Check sheet for the modelled part. Datum: model origin and axes. Units: mm. A direction names the side the tool comes from. Round coordinates to 2 decimals unless told otherwise and drop trailing zeros. Write each loop counter-clockwise with the first axis right and the second up, starting at its lowest first coordinate (ties: lowest second). Pieces come first, ordered by that corner, then holes. Notation, with made-up numbers: (59, 0) -> (105, 0) arc R3 ccw to (105, 4) -> close; hole circle Ø10 at (51.5, 17). An arc over 180 degrees is marked (long way). One line per item, written item: value.
from build123d import *
from OCP.BRepFilletAPI import BRepFilletAPI_MakeChamfer

# Parameters (mm, degrees)
SKETCH1_R           = 2.5
SKETCH1_R_2         = 3.15
BOSS_EXTRUDE1_DEPTH = 16
SKETCH2_W           = 40
SKETCH2_H           = 20
CUT_EXTRUDE1_DEPTH  = 11
FILLET2_R           = 9
SKETCH3_R           = 6
CUT_EXTRUDE2_DEPTH  = 13.5
CUT_EXTRUDE5_DEPTH  = 67.957075802
SKETCH7_R           = 3.05
CUT_EXTRUDE6_DEPTH  = 67.957075802
CHAMFER2_SIZE       = 2
CHAMFER2_SIZE2      = 0.727940469
SKETCH10_R          = 6.1
CUT_EXTRUDE8_DEPTH  = 0.7
CHAMFER3_SIZE       = 3
CHAMFER4_SIZE       = 0.3
SKETCH11_R          = 1.65
CUT_EXTRUDE9_DEPTH  = 78.111931632
SKETCH12_R          = 3.2
CUT_EXTRUDE10_DEPTH = 3
CUT_EXTRUDE11_START = -35
CUT_EXTRUDE11_DEPTH = 43.111931632
CHAMFER5_SIZE       = 2
CHAMFER5_SIZE2      = 0.727940469
CUT_EXTRUDE12_DEPTH = 78.111931632


with BuildPart() as part:
    # Sketch1 → Boss-Extrude1 (new body)
    with BuildSketch(Plane.XY):
        with BuildLine():
            Line((-61, 13.5), (-61, -12.5))
            Line((-61, -12.5), (-15, -12.5))
            Line((-15, -12.5), (1.057538487, -10.949046184))
            ThreePointArc((1.057538487, -10.949046184), (8.143491983, -7.394831866), (11, 0))
            Line((11, 0), (11, 22.5))
            Line((11, 22.5), (-26.5, 22.5))
            Line((-26.5, 22.5), (-26.5, 13.5))
            Line((-26.5, 13.5), (-61, 13.5))
        make_face()
        with Locations((-48, 0.5)):
            Circle(SKETCH1_R, mode=Mode.SUBTRACT)
        with Locations((-28, 0.5)):
            Circle(SKETCH1_R_2, mode=Mode.SUBTRACT)
    extrude(amount=BOSS_EXTRUDE1_DEPTH)

    # Sketch2 → Cut-Extrude1 (cut)
    with BuildSketch(Plane.XY.offset(16)):
        with Locations((-38, 0.5)):
            Rectangle(SKETCH2_W, SKETCH2_H)
    extrude(amount=-CUT_EXTRUDE1_DEPTH, mode=Mode.SUBTRACT)

    # Fillet2
    fillet2_edges = [part.edges().sort_by_distance(p)[0] for p in [
        (-7.75, 22.5, 0),
    ]]
    fillet(fillet2_edges, radius=FILLET2_R)

    # Sketch3 → Cut-Extrude2 (cut)
    with BuildSketch(Plane.XY.offset(16)):
        Circle(SKETCH3_R)
    extrude(amount=-CUT_EXTRUDE2_DEPTH, mode=Mode.SUBTRACT)

    # Sketch6 → Cut-Extrude5 (cut, through all)
    with BuildSketch(Plane.XY.offset(16)):
        with BuildLine():
            Line((-0.4, 24.334661422), (0.4, 24.334661422))
            Line((0.4, 24.334661422), (0.4, 2.973213749))
            ThreePointArc((0.4, 2.973213749), (0, -3), (-0.4, 2.973213749))
            Line((-0.4, 2.973213749), (-0.4, 24.334661422))
        make_face()
    extrude(amount=-CUT_EXTRUDE5_DEPTH, mode=Mode.SUBTRACT)

    # Sketch7 → Cut-Extrude6 (cut, through all)
    with BuildSketch(Plane(origin=(0, 0, 0), x_dir=(-1, 0, 0), z_dir=(0, 0, -1))):
        with Locations((48, 0.5)):
            Circle(SKETCH7_R)
    extrude(amount=-CUT_EXTRUDE6_DEPTH, mode=Mode.SUBTRACT)

    # Chamfer2: one chamfer whose edges measure the first distance from different faces: ONE call of the kernel's chamfer builder (chamfer() names one face for all edges)
    chamfer2_edges_1 = [part.edges().sort_by_distance(p)[0] for p in [
        (-58, 0.5, 16),
    ]]
    chamfer2_side_1 = [part.faces().sort_by_distance(p)[0] for p in [
        (-58, 0.5, 10.5),
    ]]
    chamfer2_edges_2 = [part.edges().sort_by_distance(p)[0] for p in [
        (-38, -9.5, 16),
    ]]
    chamfer2_side_2 = [part.faces().sort_by_distance(p)[0] for p in [
        (-38, -9.5, 10.5),
    ]]
    chamfer2_edges_3 = [part.edges().sort_by_distance(p)[0] for p in [
        (-18, 0.5, 16),
    ]]
    chamfer2_side_3 = [part.faces().sort_by_distance(p)[0] for p in [
        (-18, 0.5, 10.5),
    ]]
    chamfer2_edges_4 = [part.edges().sort_by_distance(p)[0] for p in [
        (-38, 10.5, 16),
    ]]
    chamfer2_side_4 = [part.faces().sort_by_distance(p)[0] for p in [
        (-38, 10.5, 10.5),
    ]]
    chamfer2 = BRepFilletAPI_MakeChamfer(part.part.solid().wrapped)
    for e in chamfer2_edges_1:
        chamfer2.Add(CHAMFER2_SIZE, CHAMFER2_SIZE2, e.wrapped, chamfer2_side_1[0].wrapped)  # the first distance lies on this face
    for e in chamfer2_edges_2:
        chamfer2.Add(CHAMFER2_SIZE, CHAMFER2_SIZE2, e.wrapped, chamfer2_side_2[0].wrapped)  # the first distance lies on this face
    for e in chamfer2_edges_3:
        chamfer2.Add(CHAMFER2_SIZE, CHAMFER2_SIZE2, e.wrapped, chamfer2_side_3[0].wrapped)  # the first distance lies on this face
    for e in chamfer2_edges_4:
        chamfer2.Add(CHAMFER2_SIZE, CHAMFER2_SIZE2, e.wrapped, chamfer2_side_4[0].wrapped)  # the first distance lies on this face
    add(Compound.cast(chamfer2.Shape()), mode=Mode.REPLACE)

    # Sketch10 → Cut-Extrude8 (cut)
    with BuildSketch(Plane(origin=(0, 0, 0), x_dir=(-1, 0, 0), z_dir=(0, 0, -1))):
        with Locations((28, 0.5)):
            Circle(SKETCH10_R)
        with Locations((48, 0.5)):
            Circle(SKETCH10_R)
    extrude(amount=-CUT_EXTRUDE8_DEPTH, mode=Mode.SUBTRACT)

    # Chamfer3
    # the kernel refuses this chamfer: 3 mm, written as the material it takes off along each edge
    with BuildSketch(Plane(origin=(-48, 0.5, 0.7), x_dir=(-1, 0, 0), z_dir=(0, -1, 0))) as chamfer3_piece_1:
        Polygon((3.05, -CHAMFER3_SIZE), (3.05 + CHAMFER3_SIZE, 0), (3.05, 0), align=None)
    revolve(axis=Axis((-48, 0.5, 0.7), (0, 0, -1)), mode=Mode.SUBTRACT)
    with BuildSketch(Plane(origin=(-28, 0.5, 0.7), x_dir=(1, 0, 0), z_dir=(0, 1, 0))) as chamfer3_piece_2_section:
        Polygon((3.15, -CHAMFER3_SIZE), (3.15 + CHAMFER3_SIZE, 0), (3.15, 0), align=None)
    chamfer3_piece_2 = revolve(axis=Axis((-28, 0.5, 0.7), (0, 0, -1)), mode=Mode.PRIVATE)
    chamfer3_piece_2 = chamfer3_piece_2 & Plane(origin=(-28, 0.5, 0.7), x_dir=(-1, 0, 0), z_dir=(0, 0, -1)) * Cylinder(6.1, 25, mode=Mode.PRIVATE)
    add(chamfer3_piece_2, mode=Mode.SUBTRACT)

    # Chamfer4
    # the kernel refuses this chamfer: 0.3 mm, written as the material it takes off along each edge
    with BuildSketch(Plane(origin=(0, 0, 0), x_dir=(-0.0031415874858789867, 0.9999950652018582, 0), z_dir=(0.9999950652018582, 0.0031415874858789867, 0))) as chamfer4_piece_1:
        Polygon((3 + CHAMFER4_SIZE, 0), (3, CHAMFER4_SIZE), (3, 0), align=None)
    revolve(axis=Axis((0, 0, 0), (0, 0, 1)), revolution_arc=359.64, mode=Mode.SUBTRACT)
    with BuildSketch(Plane(origin=(-61, 14.271504896, 0), x_dir=(1, 0, 0), z_dir=(0, -1, 0))) as chamfer4_piece_2:
        Polygon((CHAMFER4_SIZE, 0), (0, CHAMFER4_SIZE), (0, 0), align=None)
    extrude(amount=27.543009793, mode=Mode.SUBTRACT)
    with BuildSketch(Plane(origin=(-61.771504896, -12.5, 0), x_dir=(0, 1, 0), z_dir=(1, 0, 0))) as chamfer4_piece_3:
        Polygon((CHAMFER4_SIZE, 0), (0, CHAMFER4_SIZE), (0, 0), align=None)
    extrude(amount=50.629029378, mode=Mode.SUBTRACT)
    with BuildSketch(Plane(origin=(-18.839655792, -12.870861873, 0), x_dir=(-0.0961398624557926, 0.9953678349469514, 0), z_dir=(0.9953678349469514, 0.09613986245579259, 0))) as chamfer4_piece_4:
        Polygon((CHAMFER4_SIZE, 0), (0, CHAMFER4_SIZE), (0, 0), align=None)
    extrude(amount=19.989790287, mode=Mode.SUBTRACT)
    with BuildSketch(Plane(origin=(0, 0, 0), x_dir=(0.0961398624557928, -0.9953678349469512, 0), z_dir=(-0.9953678349469512, -0.0961398624557928, 0))) as chamfer4_piece_5:
        Polygon((11 - CHAMFER4_SIZE, 0), (11, CHAMFER4_SIZE), (11, 0), align=None)
    revolve(axis=Axis((0, 0, 0), (0, 0, 1)), revolution_arc=84.483070562, mode=Mode.SUBTRACT)
    with BuildSketch(Plane(origin=(-28, 0.5, 0), x_dir=(-1, 0, 0), z_dir=(0, -1, 0))) as chamfer4_piece_6:
        Polygon((6.1 + CHAMFER4_SIZE, 0), (6.1, -CHAMFER4_SIZE), (6.1, 0), align=None)
    revolve(axis=Axis((-28, 0.5, 0), (0, 0, -1)), mode=Mode.SUBTRACT)
    with BuildSketch(Plane(origin=(-48, 0.5, 0), x_dir=(-1, 0, 0), z_dir=(0, -1, 0))) as chamfer4_piece_7:
        Polygon((6.1 + CHAMFER4_SIZE, 0), (6.1, -CHAMFER4_SIZE), (6.1, 0), align=None)
    revolve(axis=Axis((-48, 0.5, 0), (0, 0, -1)), mode=Mode.SUBTRACT)
    with BuildSketch(Plane(origin=(0.4, 17.357524482, 0), x_dir=(1, 0, 0), z_dir=(0, -1, 0)), Plane(origin=(-0.4, 2.201708853, 0), x_dir=(-1, 0, 0), z_dir=(0, 1, 0))) as chamfer4_piece_8:
        Polygon((CHAMFER4_SIZE, 0), (0, CHAMFER4_SIZE), (0, 0), align=None)
    extrude(amount=15.155815629, mode=Mode.SUBTRACT)
    with BuildSketch(Plane(origin=(11, 0, 0), x_dir=(0, 0, 1), z_dir=(0, 1, 0))) as chamfer4_piece_9:
        Polygon((CHAMFER4_SIZE, 0), (0, -CHAMFER4_SIZE), (0, 0), align=None)
    extrude(amount=17.357524482, mode=Mode.SUBTRACT)
    with BuildSketch(Plane(origin=(-26.5, 13.5, 0), x_dir=(0, -1, 0), z_dir=(-1, 0, 0))) as chamfer4_piece_10:
        Polygon((CHAMFER4_SIZE, 0), (0, CHAMFER4_SIZE), (0, 0), align=None)
    extrude(amount=35.271504896, mode=Mode.SUBTRACT)

    # Sketch11 → Cut-Extrude9 (cut, through all)
    with BuildSketch(Plane(origin=(11, 0, 0), x_dir=(0, 0, -1), z_dir=(1, 0, 0))):
        with Locations((-9.790309274, 17.6)):
            Circle(SKETCH11_R)
    extrude(amount=-CUT_EXTRUDE9_DEPTH, mode=Mode.SUBTRACT)

    # Sketch12 → Cut-Extrude10 (cut)
    with BuildSketch(Plane(origin=(11, 0, 0), x_dir=(0, 0, -1), z_dir=(1, 0, 0))):
        with Locations((-9.790309274, 17.6)):
            Circle(SKETCH12_R)
    extrude(amount=-CUT_EXTRUDE10_DEPTH, mode=Mode.SUBTRACT)

    # Sketch13 → Cut-Extrude11 (cut, through all)
    with BuildSketch(Plane(origin=(11, 0, 0), x_dir=(0, 0, -1), z_dir=(1, 0, 0)).offset(CUT_EXTRUDE11_START)):
        Polygon((-9.386164085, 22.5), (-16, 22.5), (-16, 14.8), (-8.17372852, 14.8), (-6.557147766, 17.6), align=None)
    extrude(amount=-CUT_EXTRUDE11_DEPTH, mode=Mode.SUBTRACT)

    # Chamfer5
    chamfer5_edges = [part.edges().sort_by_distance(p)[0] for p in [
        (-4.098780306, -4.38178046, 16),
    ]]
    chamfer5_side = [part.faces().sort_by_distance(p)[0] for p in [
        (-4.098780306, -4.38178046, 9.25),
    ]]
    chamfer(chamfer5_edges, length=CHAMFER5_SIZE, length2=CHAMFER5_SIZE2, reference=chamfer5_side[0])

    # Sketch14 → Cut-Extrude12 (cut, through all)
    with BuildSketch(Plane(origin=(11, 0, 0), x_dir=(0, 0, -1), z_dir=(1, 0, 0))):
        Polygon((-9.790309274, 17.6), (-10.957035463, 18.766726189), (-11.760309274, 17.963452378), (-11.760309274, 17.236547622), (-10.957035463, 16.433273811), align=None)
    extrude(amount=-CUT_EXTRUDE12_DEPTH, mode=Mode.SUBTRACT)


solid = part.part
Item 1: Thickness scan on line 1 (X direction, y = 6.5, z = 7.25); line 2 (Y direction, x = -28, z = 4.45); line 3 (X direction, y = 15, z = 8.25). Record the ranges inside material, lowest first.
Answer:
line 1: x = -61 to -58, -18 to -0.4, 0.4 to 11
line 2: y = -12.5 to -2.65, 3.65 to 13.5
line 3: x = -24 to -0.4, 0.4 to 8
Item 2: Sectioned sample at B-B on y = 8.5. Enter the section's corners in (x, z).
Answer:
outline: (-61, 0.3) -> (-60.7, 0) -> (-0.7, 0) -> (-0.4, 0.3) -> (-0.4, 16) -> (-17.27, 16) -> (-18, 14) -> (-18, 5) -> (-58, 5) -> (-58, 14) -> (-58.73, 16) -> (-61, 16) -> close; (0.4, 0.3) -> (0.7, 0) -> (10.7, 0) -> (11, 0.3) -> (11, 16) -> (0.4, 16) -> close
Item 3: Sectioned sample at C-C on x = -37. Enter the section's corners in (y, z), and give its area (3 significant figures).
Answer:
outline: (-12.5, 0.3) -> (-12.2, 0) -> (13.2, 0) -> (13.5, 0.3) -> (13.5, 16) -> (11.23, 16) -> (10.5, 14) -> (10.5, 5) -> (-9.5, 5) -> (-9.5, 14) -> (-10.23, 16) -> (-12.5, 16) -> close
area: 194 mm^2
Item 4: Tool access check on faces 1 (the flat face through (-25.232, 16.18, 7.377)), 2 (the cylindrical face through (-53.635, -1.836, 0.497)), 3 (the flat face through (-0.4, 13, 8)), 4 (the flat face through (-38, 1, 5)), 5 (the cylindrical face through (9.52, 19.76, 12.15)). Record the directions out of +Z, -Z, +X, -X, +Y, -Y that give a thin tool (end or side, any length) a straight path to the whole face; none if there is none.
Answer:
face 1: +Z, -X
face 2: -Z
face 3: +Z, -Z, +Y
face 4: +Z
face 5: +X
Item 5: Depth check by flat-ended pin: P1, Ø1, axis at y = 15, z = 3, coming from the -X side; P2, Ø1.5, axis at y = -1.5, z = 4.5, coming from the +X side; P3, Ø10, axis at x = -29, y = -4, coming from the +Z side. Enter the tip coordinate at first touch or a pass-through.
Answer:
P1: stops at x = -26.5
P2: stops at x = 10.97
P3: stops at z = 5
Item 6: Mould release check, pull along X, two halves, no side actions. Record for faces 6 (the flat face through (-26.5, 17, 6)), 7 (the cylindrical face through (4.25, 17.55, 8.14)), 8 (the flat face through (-38.29, -9.869, 15.014)): pulls with the +X half, pulls with the -X half, needs draft (parallel to the pull), parting line crosses it, or undercut.
Answer:
face 6: pulls with the -X half
face 7: needs draft
face 8: undercut
Item 7: Sectioned sample at A-A on x = -48. Enter the section's corners in (y, z), and give its area (3 significant figures).
Answer:
outline: (-12.5, 0.3) -> (-12.2, 0) -> (-5.9, 0) -> (-5.6, 0.3) -> (-5.6, 0.7) -> (-5.55, 0.7) -> (-2.55, 3.7) -> (-2.55, 5) -> (-9.5, 5) -> (-9.5, 14) -> (-10.23, 16) -> (-12.5, 16) -> close; (3.55, 3.7) -> (6.55, 0.7) -> (6.6, 0.7) -> (6.6, 0.3) -> (6.9, 0) -> (13.2, 0) -> (13.5, 0.3) -> (13.5, 16) -> (11.23, 16) -> (10.5, 14) -> (10.5, 5) -> (3.55, 5) -> close
area: 151 mm^2
Item 8: Sectioned sample at D-D on x = -28. Enter the section's corners in (y, z), and give its area (3 significant figures).
Answer:
outline: (-12.5, 0.3) -> (-12.2, 0) -> (-5.9, 0) -> (-5.6, 0.3) -> (-5.6, 0.75) -> (-2.65, 3.7) -> (-2.65, 5) -> (-9.5, 5) -> (-9.5, 14) -> (-10.23, 16) -> (-12.5, 16) -> close; (3.65, 3.7) -> (6.6, 0.75) -> (6.6, 0.3) -> (6.9, 0) -> (13.2, 0) -> (13.5, 0.3) -> (13.5, 16) -> (11.23, 16) -> (10.5, 14) -> (10.5, 5) -> (3.65, 5) -> close
area: 150 mm^2
